Source: CAD feature listing. Evaluate the final solid. Frame: model axes, mm. Face numbers are marked on the shaded views. A direction names the side the tool comes from. Give positions to 0.01 mm unless a question says otherwise; leave off trailing zeros. Write each loop counter-clockwise with the first axis right and the second up, starting at its lowest first coordinate (ties: lowest second). Pieces come first, ordered by that corner, then holes. Notation, with made-up numbers: (-37.5, -7) - (-1.5, -7) arc R19 cw to (-1.5, 16) - close; hole circle Ø10 at (12.5, 57.25). An arc over 180 degrees is marked (long way). One line per question, with ' | ' between items. Start each with the question number.
(1) Pin query (flat end, axial travel): pin 1 (8 mm diameter, centred on x = 0, y = 5, fed in from +Z); pin 2 (2.5 mm diameter, centred on x = 0, y = 5, fed in from -Z); pin 3 (3 mm diameter, centred on x = 0, y = 4.5, fed in from +Z). Return the tip coordinate at first contact, or that it passes through.
(2) Section C-C, the plane x = -6.25. Return loops of the section in (y, z), plus the area to 3 significant figures.
(3) Section D-D, the plane z = 1.5. Return loops of the section in (x, y), plus the area to 3 significant figures.
(4) Ray query, line 1 (Z direction, x = -4.5, y = 8.75); line 2 (Y direction, x = 0, z = 14.45); line 3 (Y direction, x = 0, z = 11.15). Return the intervals inside material, ascending. Write a range as [from, to].
(5) Section A-A, the plane y = 5. Return loops of the section in (x, z), plus the area to 3 significant figures.
(6) Access query for the marked faces 1 and 2. Directions: +Z, -Z, +X, -X, +Y, -Y. A direction counts if a zero-diameter tool reaches every point of the face in a straight line with its end or side. Return the directions, or none.
(7) Section B-B, the plane z = 12.5. Return loops of the section in (x, y), plus the area to 3 significant figures.
(8) Draft query along X for the marked faces 3, 4, 5 and 6. Return one class per face: +X half, -X half, draft (parallel to the pull), parting line (faces both ways), or undercut.
```python
from build123d import *

# Parameters (mm, degrees)
SKETCH1_W           = 30
SKETCH1_H           = 30
BOSS_EXTRUDE1_DEPTH = 15
SKETCH2_W           = 20
SKETCH2_H           = 20
CUT_EXTRUDE1_DEPTH  = 10
SKETCH3_R           = 1.5
CUT_EXTRUDE2_DEPTH  = 30
CUT_EXTRUDE3_DEPTH  = 2
SKETCH5_R           = 3
CUT_EXTRUDE4_DEPTH  = 2


with BuildPart() as part:
    # Sketch1 → Boss-Extrude1 (new body)
    with BuildSketch(Plane(origin=(0, 0, 0), x_dir=(1, 0, 0), z_dir=(0, 1, 0))):
        Rectangle(SKETCH1_W, SKETCH1_H)
    extrude(amount=BOSS_EXTRUDE1_DEPTH)

    # Sketch2 → Cut-Extrude1 (cut)
    with BuildSketch(Plane.XZ):
        Rectangle(SKETCH2_W, SKETCH2_H)
    extrude(amount=-CUT_EXTRUDE1_DEPTH, mode=Mode.SUBTRACT)

    # Sketch3 → Cut-Extrude2 (cut)
    with BuildSketch(Plane(origin=(0, 0, -15), x_dir=(-1, 0, 0), z_dir=(0, 0, -1))):
        with Locations((0, 5)):
            Circle(SKETCH3_R)
    extrude(amount=-CUT_EXTRUDE2_DEPTH, mode=Mode.SUBTRACT)

    # Sketch4 → Cut-Extrude3 (cut)
    with BuildSketch(Plane(origin=(0, 0, -15), x_dir=(-1, 0, 0), z_dir=(0, 0, -1))):
        Polygon((0, 2.070756219), (2.536799528, 3.53537811), (2.536799528, 6.46462189), (0, 7.929243781), (-2.536799528, 6.46462189), (-2.536799528, 3.53537811), align=None)
    extrude(amount=-CUT_EXTRUDE3_DEPTH, mode=Mode.SUBTRACT)

    # Sketch5 → Cut-Extrude4 (cut)
    with BuildSketch(Plane.XY.offset(15)):
        with Locations((0, 5)):
            Circle(SKETCH5_R)
    extrude(amount=-CUT_EXTRUDE4_DEPTH, mode=Mode.SUBTRACT)


solid = part.part
```
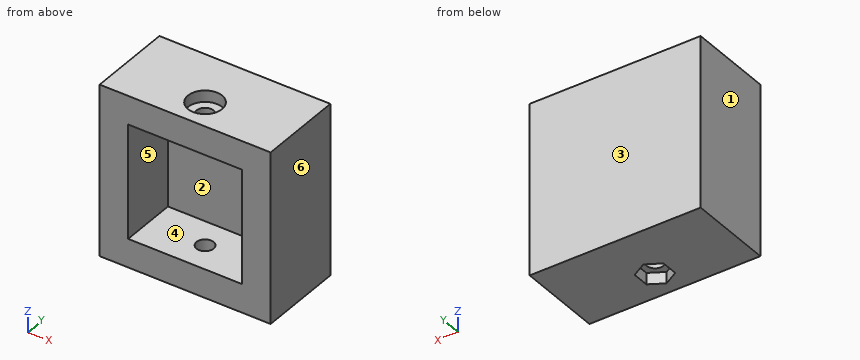
Check sheet entries:
1) pin 1: z = 15 | pin 2: through | pin 3: z = 13
2) outline: (0, -15) - (15, -15) - (15, 15) - (0, 15) - (0, 10) - (10, 10) - (10, -10) - (0, -10) - close | area: 250 mm²
3) outline: (-15, 0) - (-10, 0) - (-10, 10) - (10, 10) - (10, 0) - (15, 0) - (15, 15) - (-15, 15) - close | area: 250 mm²
4) line 1: [-15, -10], [10, 15] | line 2: [0, 2], [8, 15] | line 3: [0, 3.5], [6.5, 15]
5) outline: (-15, -15) - (-2.54, -15) - (-2.54, -13) - (-1.5, -13) - (-1.5, -10) - (-10, -10) - (-10, 10) - (-1.5, 10) - (-1.5, 13) - (-3, 13) - (-3, 15) - (-15, 15) - close; (1.5, -13) - (2.54, -13) - (2.54, -15) - (15, -15) - (15, 15) - (3, 15) - (3, 13) - (1.5, 13) - (1.5, 10) - (10, 10) - (10, -10) - (1.5, -10) - close | area: 460 mm²
6) face 1: +Z, -Z, -X, +Y, -Y | face 2: -Y
7) outline: (-15, 0) - (15, 0) - (15, 15) - (-15, 15) - close; hole circle Ø3 at (0, 5) | area: 443 mm²
8) face 3: draft | face 4: undercut | face 5: undercut | face 6: +X half
